Autodesk Inventor part; units mm, degrees
ref_plane "YZ Plane" through (0, 0, 0) normal (1, 0, 0) x (0, 1, 0)
ref_plane "XZ Plane" through (0, 0, 0) normal (0, 1, 0) x (-1, 0, 0)
ref_plane "XY Plane" through (0, 0, 0) normal (0, 0, 1) x (1, 0, 0)
sketch "Эскиз5" plane through (0, 0, 0) normal (0, 0, 1) x (1, 0, 0)
  line L0 (0, 0) -> (20, 0)
  line L1 (20, 0) -> (20, 25)
  line L2 (16, 29) -> (4, 29)
  line L3 (0, 25) -> (0, 0)
  line L4 (4, 29) -> (0, 25)
  line L5 (16, 29) -> (20, 25)
  point P0 (20, 29)
  point P1 (0, 29)
  dimension "d25" = 20
  dimension "d26" = 29
  dimension "d27" = 4
  dimension "d28" = 4
  dimension "d29" = 4
  dimension "d30" = 4
revolve "Вращение3" add sketch "Эскиз5" angle 360 about axis through (0, 0, 0) along (1, 0, 0)
sketch "Эскиз6" plane through (20, 0, 0) normal (1, 0, 0) x (0, 0, -1)
  point P0 (0, 0)
  point P1 (0, 0)
hole "Отверстие2" at (20, 0, 0) direction (-1, 0, 0) diameter 10 depth 5
sketch "Эскиз7" plane through (15, 0, 0) normal (1, 0, 0) x (0, 0, -1)
  point P0 (0, 0)
  point P1 (0, 0)
hole "Отверстие3" at (15, 0, 0) direction (-1, 0, 0) diameter 5 depth 3
sketch "Эскиз8" plane through (0, 0, 0) normal (0, 0, 1) x (1, 0, 0)
  line L0 (20, -25) -> (20, 25) construction
  line L1 (20, 25) -> (16, 25)
  line L2 (16, 25) -> (16, 21.5)
  line L3 (16, 21.5) -> (20, 21.5)
  line L4 (20, 21.5) -> (20, 25)
  line L5 (0, 0) -> (20, 0)
  dimension "d46" = 4
  dimension "d47" = 3.5
revolve "Вращение4" cut sketch "Эскиз8" angle 360 about axis through (0, 0, 0) along (1, 0, 0)
sketch "Эскиз9" plane through (0, 0, 0) normal (0, 0, 1) x (1, 0, 0)
  line L0 (0, -25) -> (0, 25) construction
  line L1 (0, 4) -> (9, 4)
  line L2 (9, 4) -> (9, -4)
  line L3 (9, -4) -> (0, -4)
  line L4 (0, -4) -> (0, 4)
  point P0 (0, 0)
  point P1 (0, 0)
  point P2 (0, 0)
  dimension "d49" = 9
  dimension "d50" = 8
extrude "Выдавливание2" cut sketch "Эскиз9" along normal through all both and the other way through all
sketch "Эскиз10" plane through (0, 0, 0) normal (-1, 0, 0) x (0, 0, 1)
  line L0 (0, 0) -> (0, 20) construction
  dimension "d53" = 20
hole "Отверстие4" at (0, 20, 0) direction (1, 0, 0) diameter 4 depth 4 tip angle 118
properties part number "711128"
Part model, mm, in its own coordinate system. A direction names the side the tool comes from. Coordinates: 2 decimals unless noted, no trailing zeros. Loops run counter-clockwise (first coordinate to the right, second up) from the corner with the lowest first, then second, coordinate; pieces in that order, holes last. Notation, with made-up numbers: (-31, 83) -> (-27, 83) arc R28 cw to (-27, 117) -> close; hole circle Ø8 at (10, 52). An arc over 180 degrees is marked (long way). Use a Markdown table: item, result. Add a question column.
Item 1: Band-saw the part on A-A on x = 17. Write the cut outline in (y, z).
Item 2: Pull direction Y, two halves, no side cores. Call faces 1 (the cylindrical face through (2, 18, 0)), 2 (the conical face through (0.25, -25.245, 0.506)), 3 (the flat face through (20, 4, -4)): +Y half, -Y half, draft (parallel to the pull), parting line (faces both ways), or undercut.
Item 3: Probe probe 1 along Y at (x, z) = (3.75, 0); probe 2 along Z at (x, y) = (12.85, 0); probe 3 along Y at (x, z) = (1.35, 0). List the from-to ranges inside material, lowest first.
Item 4: Band-saw the part on B-B on y = 0. Write the cut outline in (x, z).
Item 5: Which spindle directions (+Z, -Z, +X, -X, +Y, -Y) get a long thin tool onto all of the face, cutting with end or side? Do faces 4 (the flat face through (16, 11, 19)), 5 (the flat face through (0, -12, 0)), 6 (the flat face through (9, 0, 0)). Say none if no direction does.
Item 6: Flat gauge pins, fed straight in: P1, Ø12, axis at x = 11.5, z = -19, coming from the -Y side; P2, Ø5, axis at x = 9.5, z = 20.5, coming from the +Y side; P3, Ø8, axis at x = 15, y = -8, coming from the -Z side; P4, Ø7, axis at x = 4.5, z = 1, coming from the -Y side. Where does each tip first touch, or does it go through?
Geometry says:
| question | item | result |
|---|---|---|
| 1 | outline | circle Ø56 at (0, 0); circle Ø43 at (0, 0); hole circle Ø50 at (0, 0); hole circle Ø10 at (0, 0) |
| 2 | face 1 | undercut |
| 2 | face 2 | -Y half |
| 2 | face 3 | draft |
| 3 | probe 1 | -28.75 to -4, 4 to 18, 22 to 28.75 |
| 3 | probe 2 | -29 to -2.5, 2.5 to 29 |
| 3 | probe 3 | -26.35 to -4, 4 to 18, 22 to 26.35 |
| 4 | outline | (9, -29) -> (16, -29) -> (20, -25) -> (16, -25) -> (16, -21.5) -> (20, -21.5) -> (20, -5) -> (15, -5) -> (15, -2.5) -> (12, -2.5) -> (12, 2.5) -> (15, 2.5) -> (15, 5) -> (20, 5) -> (20, 21.5) -> (16, 21.5) -> (16, 25) -> (20, 25) -> (16, 29) -> (9, 29) -> close |
| 5 | face 4 | +X |
| 5 | face 5 | +Z, -Z, -X, +Y, -Y |
| 5 | face 6 | +Z, -Z, -X |
| 6 | P1 | y = -25.92 |
| 6 | P2 | y = 22.74 |
| 6 | P3 | z = -28.72 |
| 6 | P4 | y = -29 |
